Can you work these out from the model? Positions are in its coordinate system, mm. A direction names the side the tool comes from. Give positions to 0.01 mm unless a question says otherwise; leave off trailing zeros. Order: outer loops, then holes, each group sorted by start corner. A loop starts at its lowest first (then second) coordinate and runs counter-clockwise, first axis right, second up. Notation, with made-up numbers: (37.25, -29.5) - (84.25, -29.5) arc R34 ccw to (84.25, 0.5) - close; hole circle Ø1 at (-22, 38). An arc over 180 degrees is marked (long way). Return JSON: item names as keys, results as strings.
```python
from build123d import *

# Parameters (mm, degrees)
SKETCH_1_R               = 60
EXTRUDE_1_DEPTH          = 8
FILLET_1_R               = 100
EXTRUDE_START            = 10
EXTRUDE_2_DEPTH          = 10
FILLET_2_R               = 10
CHAMFER_1_SIZE           = 5
CUT_EXTRUDE_1_DEPTH      = 434.442567426
CUT_EXTRUDE_1_DEPTH_BACK = 434.442567426
SKETCH_3_R               = 4.3


with BuildPart() as part:
    # 草图1 → 凸台-拉伸1 (new body)
    with BuildSketch(Plane.XY):
        Polygon((0, 0), (0, 280), (861.751390409, 0), align=None)
        with Locations((200, 100)):
            Circle(SKETCH_1_R, mode=Mode.SUBTRACT)
    extrude(amount=EXTRUDE_1_DEPTH)

    # 圆角1
    fillet_1_edges = [part.edges().sort_by_distance(p)[0] for p in [
        (861.751390409, 0, 4),
    ]]
    fillet(fillet_1_edges, radius=FILLET_1_R)

    # 草图2 → 凸台-拉伸2 (add)
    with BuildSketch(Plane.XY.offset(8).offset(EXTRUDE_START)):
        with BuildLine():
            Line((0, 0), (230.376238942, 0))
            ThreePointArc((230.376238942, 0), (329.145073001, 84.356553496), (261.277938379, 195.10565163))
            Line((261.277938379, 195.10565163), (0, 280))
            Line((0, 280), (0, 0))
        make_face()
        Polygon((10, 266.236180795), (10, 35.358983849), (122.241374643, 229.766747442), align=None, mode=Mode.SUBTRACT)
        with BuildLine():
            Line((30, 10), (230.376238942, 10))
            ThreePointArc((230.376238942, 10), (319.268189595, 85.920898146), (258.187768435, 185.595086467))
            Line((258.187768435, 185.595086467), (151.410485182, 220.289128906))
            Line((151.410485182, 220.289128906), (30, 10))
        make_face(mode=Mode.SUBTRACT)
    extrude(amount=-EXTRUDE_2_DEPTH)

    # 圆角2
    fillet_2_edges = [part.edges().sort_by_distance(p)[0] for p in [
        (10, 266.236180795, 13),
        (10, 35.358983849, 13),
        (122.241374643, 229.766747442, 13),
        (30, 10, 13),
        (151.410485182, 220.289128906, 13),
    ]]
    fillet(fillet_2_edges, radius=FILLET_2_R)

    # 倒角1
    chamfer_1_edges = [part.edges().sort_by_distance(p)[0] for p in [
        (130.63896919, 237.552825815, 0),
        (329.145073001, 84.356553496, 0),
        (115.188119471, 0, 18),
        (329.145073001, 84.356553496, 18),
        (130.63896919, 237.552825815, 18),
        (115.188119471, 0, 0),
    ]]
    chamfer(chamfer_1_edges, length=CHAMFER_1_SIZE)

    # 草图3 → 切除-拉伸1 (cut, two sides: drawn at the far end of the back side and taken through both)
    with BuildSketch(Plane(origin=(0, 0, 0), x_dir=(-1, 0, 0), z_dir=(0, 0, -1)).offset(-CUT_EXTRUDE_1_DEPTH_BACK)):
        with Locations((-64, 217)):
            Circle(SKETCH_3_R)
        with Locations((-64, 177)):
            Circle(SKETCH_3_R)
        with Locations((-24, 217)):
            Circle(SKETCH_3_R)
        with Locations((-24, 177)):
            Circle(SKETCH_3_R)
        with Locations((-64, 89)):
            Circle(SKETCH_3_R)
        with Locations((-24, 89)):
            Circle(SKETCH_3_R)
        with Locations((-64, 49)):
            Circle(SKETCH_3_R)
        with Locations((-24, 49)):
            Circle(SKETCH_3_R)
    extrude(amount=CUT_EXTRUDE_1_DEPTH + CUT_EXTRUDE_1_DEPTH_BACK, mode=Mode.SUBTRACT)


solid = part.part
```
1. Thinking about a two-plate mould opening in X: for faces 1 (the face through (61.688, 92.626, 9.126)), 2 (the face through (129, 112, 0)), 3 (the face through (131.71, 234.61, 15.47)), which applies, +X half, -X half, draft (parallel to the pull), parting line (faces both ways), or undercut?
Checks:
{"face 1": "undercut", "face 2": "draft", "face 3": "+X half"}
2. Suppose I cut it at C-C (y = 100). List the corners of the cut face in (x, z) for me.
Checks:
{"outline": "(0, 0) - (140, 0) - (140, 8) - (81.96, 8) - (81.96, 18) - (47.32, 18) - (47.32, 8) - (10, 8) - (10, 18) - (0, 18) - close; (260, 0) - (325.38, 0) - (330.38, 5) - (330.38, 13) - (325.38, 18) - (320.38, 18) - (320.38, 8) - (260, 8) - close"}
3. Suppose I cut it at B-B (x = 64). State how many separate pieces and enclosed holes the cut face has, plus the area to 3 significant figures.
Checks:
{"separate pieces": "5", "enclosed holes": "0", "area": "2,470 mm^2"}
4. On a 3-axis mill with a long thin cutter (end or side, diameter ignored), from which of +Z, -Z, +X, -X, +Y, -Y can I reach the whole of each face in a straight line? I mean faces 4 (the face through (22.016, 213.185, 4.056)), 5 (the face through (116.8, 227.5, 12.9)). Say none if no direction works.
Checks:
{"face 4": "+Z, -Z", "face 5": "+Z"}
5. For pin 1 Ø7.5 at (x, y) = (24, 49) entering from +Z; pin 2 Ø10 at (x, y) = (64, 217) entering from +Z; pin 3 Ø2 at (x, z) = (112, 7.5) entering from +Y; pin 4 Ø5 at (y, z) = (143, 9.5) entering from +X, each with a flat end and sliding along its axis, tell me the tip position at first contact or that it passes through.
Checks:
{"pin 1": "through", "pin 2": "z = 8", "pin 3": "y = 243.93", "pin 4": "x = 321.81"}
6. Suppose I cut it at A-A (x = 200). List the corners of the cut face in (y, z) for me, plus the area to 3 significant figures.
Checks:
{"outline": "(0, 5) - (5, 0) - (40, 0) - (40, 8) - (10, 8) - (10, 18) - (5, 18) - (0, 13) - close; (160, 0) - (209.76, 0) - (215.02, 5) - (215.02, 13) - (209.76, 18) - (204.5, 18) - (204.5, 8) - (160, 8) - close", "area": "914 mm^2"}
7. If I drill on L1, parallel to Y at x = 64, z = 3.5; L2, parallel to X at y = 89, z = 5; L3, parallel to Y at x = 22, z = 6, over which ranges is the centre line in solid material (lowest first)? Write a range as [from, to].
Checks:
{"L1": "[1.5, 44.7], [53.3, 84.7], [93.3, 172.7], [181.3, 212.7], [221.3, 257.63]", "L2": "[0, 19.7], [28.3, 59.7], [68.3, 141.02], [258.98, 329.77]", "L3": "[0, 45.19], [52.81, 85.19], [92.81, 173.19], [180.81, 213.19], [220.81, 272.85]"}
